from build123d import *

# Parameters (mm, degrees)
BOSS_EXTRUDE1_DEPTH = 31
SKETCH2_W           = 5.5
SKETCH2_H           = 10.5
CUT_EXTRUDE1_DEPTH  = 7.5
SKETCH3_R           = 3
CUT_EXTRUDE2_DEPTH  = 7.5
CUT_EXTRUDE5_REACH  = 8.5
SKETCH6_W           = 8
SKETCH6_H           = 13
FILLET1_R           = 0.5
FILLET2_R           = 4
CUT_EXTRUDE7_REACH  = 27.5
SKETCH9_R           = 1.5
CUT_EXTRUDE8_DEPTH  = 17
CUT_EXTRUDE9_DEPTH  = 10
FILLET3_R           = 5
SKETCH11_W          = 15
SKETCH11_H          = 4.374689329
CUT_EXTRUDE10_DEPTH = 7.5


with BuildPart() as part:
    # Sketch1 → Boss-Extrude1 (new body)
    with BuildSketch(Plane.XY):
        with BuildLine():
            Line((-3.75, 29), (-3.75, 22.5))
            Line((-3.75, 22.5), (-3.75, -22.5))
            Line((-3.75, -22.5), (2.75, -22.5))
            Line((2.75, -22.5), (2.75, 22.5))
            ThreePointArc((2.75, 22.5), (0.846194078, 27.096194078), (-3.75, 29))
        make_face()
    extrude(amount=BOSS_EXTRUDE1_DEPTH)

    # Sketch2 → Cut-Extrude1 (cut, through all)
    with BuildSketch(Plane.ZY.offset(3.75)):
        with Locations((28.25, 23.75)):
            Rectangle(SKETCH2_W, SKETCH2_H)
    extrude(amount=-CUT_EXTRUDE1_DEPTH, mode=Mode.SUBTRACT)

    # Sketch3 → Cut-Extrude2 (cut, through all)
    with BuildSketch(Plane.ZY.offset(3.75)):
        with Locations((21, 9)):
            Circle(SKETCH3_R)
        with Locations((21, -12.5)):
            Circle(SKETCH3_R)
    extrude(amount=-CUT_EXTRUDE2_DEPTH, mode=Mode.SUBTRACT)

    # Sketch6 → Cut-Extrude5 (cut, up to next)
    with BuildSketch(Plane.ZY.offset(3.75), mode=Mode.PRIVATE) as cut_extrude5_sk1:
        with Locations((4, 2)):
            Rectangle(SKETCH6_W, SKETCH6_H)
    cut_extrude5_tool1 = extrude(cut_extrude5_sk1.sketch, amount=-CUT_EXTRUDE5_REACH, mode=Mode.PRIVATE) & part.part
    add(cut_extrude5_tool1.solids().sort_by_distance((-3.75, 2, 4))[0], mode=Mode.SUBTRACT)

    # Fillet1
    fillet1_edges = [part.edges().sort_by_distance(p)[0] for p in [
        (-0.5, 8.5, 8),
        (-0.5, -4.5, 8),
    ]]
    fillet(fillet1_edges, radius=FILLET1_R)

    # Fillet2
    fillet2_edges = [part.edges().sort_by_distance(p)[0] for p in [
        (-0.5, -4.5, 0),
        (-0.5, 8.5, 0),
    ]]
    fillet(fillet2_edges, radius=FILLET2_R)

    # Sketch8 → Cut-Extrude7 (cut, up to next)
    with BuildSketch(Plane.XY.offset(25.5), mode=Mode.PRIVATE) as cut_extrude7_sk1:
        with BuildLine():
            Line((-3.75, 26.5), (-3.75, 18.5))
            ThreePointArc((-3.75, 18.5), (0.25, 22.5), (-3.75, 26.5))
        make_face()
    cut_extrude7_tool1 = extrude(cut_extrude7_sk1.sketch, amount=-CUT_EXTRUDE7_REACH, mode=Mode.PRIVATE) & part.part
    add(cut_extrude7_tool1.solids().sort_by_distance((-2.052347, 22.5, 25.5))[0], mode=Mode.SUBTRACT)

    # Sketch9 → Cut-Extrude8 (cut)
    with BuildSketch(Plane(origin=(0, 14.627294401, -2.055732165), x_dir=(-1, 0, 0), z_dir=(0, 0.990268069, -0.139173101))):
        with Locations((0.25, 29.426538121)):
            Circle(SKETCH9_R)
    extrude(amount=-CUT_EXTRUDE8_DEPTH, mode=Mode.SUBTRACT)

    # Sketch10 → Cut-Extrude9 (cut)
    with BuildSketch(Plane.ZY.offset(3.75)):
        Polygon((8, -7.48664609), (35.202378245, -7.48664609), (35.202378245, -24.00834186), (-1.764970627, -24.00834186), (-1.764970627, -2.884142505), (8, -2.884142505), align=None)
    extrude(amount=-CUT_EXTRUDE9_DEPTH, mode=Mode.SUBTRACT)

    # Fillet3
    fillet3_edges = [part.edges().sort_by_distance(p)[0] for p in [
        (-0.5, -7.48664609, 31),
    ]]
    fillet(fillet3_edges, radius=FILLET3_R)

    # Sketch11 → Cut-Extrude10 (cut, through all)
    with BuildSketch(Plane.ZY.offset(3.75)):
        with Locations((19.5, -0.299301426)):
            Rectangle(SKETCH11_W, SKETCH11_H)
    extrude(amount=-CUT_EXTRUDE10_DEPTH, mode=Mode.SUBTRACT)


solid = part.part
Part model, mm, in its own coordinate system. A direction names the side the tool comes from. Coordinates: 2 decimals unless noted, no trailing zeros. Write each loop counter-clockwise with the first axis right and the second up, starting at its lowest first coordinate (ties: lowest second). Pieces come first, ordered by that corner, then holes. Notation, with made-up numbers: (-22, 9) - (32, 9) arc R21 ccw to (32, 28) - close; hole circle Ø11 at (89, 71). An arc over 180 degrees is marked (long way). Put each result on its own line as item: value.
1. Flat gauge pins, fed straight in: pin 1 Ø2 at (x, z) = (-2, 6.5) entering from +Y; pin 2 Ø1.8 at (x, z) = (-1.5, 5.5) entering from -Y; pin 3 Ø2 at (x, y) = (-2, -0.5) entering from -Z. Where does each tip first touch, or does it go through?
Final values:
pin 1: stops at y = 28.96
pin 2: stops at y = 8.5
pin 3: stops at z = 8
2. Band-saw the part on D-D (x = 2.25). Write the cut outline in (y, z), then the cut area to 3 significant figures.
Final values:
outline: (-7.49, 8) - (8, 8) arc R0.5 cw to (8.5, 7.5) - (8.5, 4) arc R4 ccw to (12.5, 0) - (25, 0) - (25, 25.5) - (18.5, 25.5) - (18.5, 31) - (-2.49, 31) arc R5 ccw to (-7.49, 26) - close; hole (-2.49, 12) - (1.89, 12) - (1.89, 27) - (-2.49, 27) - close; hole circle Ø6 at (9, 21)
area: 741 mm²
3. Band-saw the part on B-B (x = -0.75). Write the cut outline in (y, z).
Final values:
outline: (-7.49, 8) - (8, 8) arc R0.5 cw to (8.5, 7.5) - (8.5, 4) arc R4 ccw to (12.5, 0) - (19.85, 0) - (19.85, 25.5) - (18.5, 25.5) - (18.5, 25.69) - (1.69, 28.05) - (2.08, 30.85) - (18.5, 28.54) - (18.5, 31) - (-2.49, 31) arc R5 ccw to (-7.49, 26) - close; (25.15, 0) - (28.27, 0) - (28.27, 25.5) - (25.15, 25.5) - close; hole (-2.49, 12) - (1.89, 12) - (1.89, 27) - (-2.49, 27) - close; hole circle Ø6 at (9, 21)
4. Two-plate mould, pull along Z, no slides. Class faces 6 (the flat face through (-0.23, 1.89, 29.47)), 7 (the cylindrical face through (-0.45, -6.06, 29.5)), 8 (the cylindrical face through (-0.454, 9.641, 1.203)), 9 (the flat face through (-1, 0, 27)): +Z half, -Z half, draft (parallel to the pull), parting line (faces both ways), or undercut.
Final values:
face 6: undercut
face 7: +Z half
face 8: -Z half
face 9: undercut
5. 3-axis set-ups, long thin cutter, end or side, ignore diameter. For faces 1 (the flat face through (-1, 1.888, 19)), 2 (the cylindrical face through (0.25, 22.41, 12.93)), 3 (the flat face through (-1, 0, 8)), 4 (the flat face through (-1, 18.5, 29)), 5 (the flat face through (-1, 8, 31)): which of +Z, -Z, +X, -X, +Y, -Y reach the whole face in a straight line?
Final values:
face 1: +X, -X
face 2: +Z, -Z, -X
face 3: -Z, +X, -X, -Y
face 4: +Z, +X, -X, +Y
face 5: +Z, +X, -X, +Y, -Y
6. Probe line 1 along Y through (x, z) = (1.5, 21); line 2 along Y through (x, z) = (-1.75, 21); line 3 along Y through (x, z) = (-2.25, 14). List the from-to ranges inside material, lowest first. Write a range as [from, to].
Final values:
line 1: y = [-7.49, -2.49], [1.89, 6], [12, 26.33]
line 2: y = [-7.49, -2.49], [1.89, 6], [12, 19.04], [25.96, 28.68]
line 3: y = [-7.49, -2.49], [1.89, 18.79], [26.21, 28.82]
7. Band-saw the part on A-A (z = 21). Write the cut outline in (x, y), then the cut area to 3 significant figures.
Final values:
outline: (-3.75, -7.49) - (2.75, -7.49) - (2.75, -2.49) - (-3.75, -2.49) - close; (-3.75, 1.89) - (2.75, 1.89) - (2.75, 6) - (-3.75, 6) - close; (-3.75, 12) - (2.75, 12) - (2.75, 22.5) arc R6.5 ccw to (-3.75, 29) - (-3.75, 26.5) arc R4 cw to (-3.75, 18.5) - close
area: 136 mm²
8. Band-saw the part on C-C (z = 15). Write the cut outline in (x, y), then the cut area to 3 significant figures.
Final values:
outline: (-3.75, -7.49) - (2.75, -7.49) - (2.75, -2.49) - (-3.75, -2.49) - close; (-3.75, 1.89) - (2.75, 1.89) - (2.75, 22.5) arc R6.5 ccw to (-3.75, 29) - (-3.75, 26.5) arc R4 cw to (-3.75, 18.5) - close
area: 175 mm²
